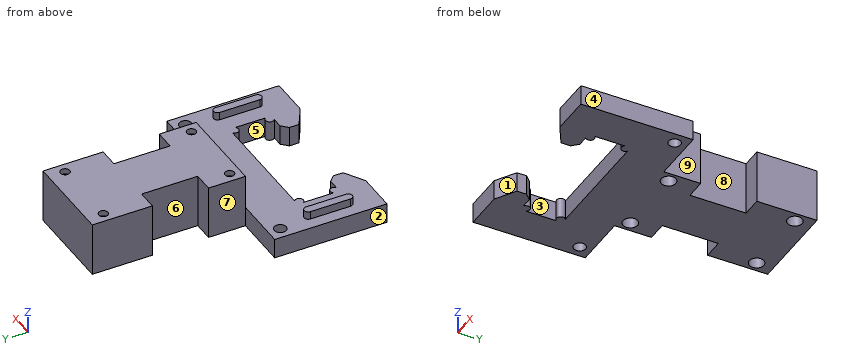
from build123d import *

# Parameters (mm, degrees)
ESQUISSE1_W             = 63.5
ESQUISSE1_H             = 35.56
BOSS_EXTRU_1_DEPTH      = 6.35
BOSS_EXTRU_2_DEPTH      = 2.54
EMPREINTE1_DEPTH        = 6.35
D_PLACER_LA_FACE2_DEPTH = 6.35
CHANFREIN1_SIZE         = 6.35
CHANFREIN1_SIZE2        = 3.81
CHANFREIN2_SIZE         = 6.35
CHANFREIN2_SIZE2        = 3.81
ESQUISSE3_W             = 29
ESQUISSE3_H             = 17.046330794
BOSS_EXTRU_3_DEPTH      = 48.514
ESQUISSE4_R             = 2.341041465
ENL_V_MAT_EXTRU_1_DEPTH = 15.24
ESQUISSE5_R             = 1.397
ESQUISSE5_W             = 6.35
ESQUISSE5_H             = 17.78
ENL_V_MAT_EXTRU_2_DEPTH = 78.134580407
D_GAGEMENT_M2_51_D      = 2.9
D_GAGEMENT_61_D         = 3.7973


# Read off the part's stored shape, not the designer's step: Empreinte1, Déplacer la face2
with BuildPart() as part:
    # Esquisse1 → Boss.-Extru.1 (new body)
    with BuildSketch(Plane.XY):
        with Locations((0, 1.905)):
            Rectangle(ESQUISSE1_W, ESQUISSE1_H)
    extrude(amount=BOSS_EXTRU_1_DEPTH)

    # Esquisse2 → Boss.-Extru.2 (add)
    with BuildSketch(Plane.XY.offset(6.35)):
        with BuildLine():
            Line((-27.94, -6.35), (-27.94, 6.35))
            ThreePointArc((-27.94, 6.35), (-26.67, 7.62), (-25.4, 6.35))
            Line((-25.4, 6.35), (-25.4, -6.35))
            ThreePointArc((-25.4, -6.35), (-26.67, -7.62), (-27.94, -6.35))
        make_face()
    boss_extru_2 = extrude(amount=BOSS_EXTRU_2_DEPTH)

    # Symétrie1: Boss.-Extru.2 across plane
    add(boss_extru_2.mirror(Plane(origin=(0, 0, 0), x_dir=(0, 0, 1), z_dir=(1, 0, 0))))

    # Empreinte1 outline → Empreinte1 (cut)
    with BuildSketch(Plane.XY):
        with BuildLine():
            Line((-11.90625, -8.5725), (-11.90625, -15.875))
            Line((-11.90625, -15.875), (11.90625, -15.875))
            Line((11.90625, -15.875), (11.90625, -8.5725))
            Line((11.90625, -8.5725), (14.44625, -6.0325))
            Line((14.44625, -6.0325), (16.66875, -6.0325))
            ThreePointArc((16.66875, -6.0325), (17.366201977, -4.348701977), (19.05, -3.65125))
            Line((19.05, -3.65125), (19.05, 2.69875))
            ThreePointArc((19.05, 2.69875), (17.366201977, 3.396201977), (16.66875, 5.08))
            Line((16.66875, 5.08), (-16.66875, 5.08))
            ThreePointArc((-16.66875, 5.08), (-17.366201977, 3.396201977), (-19.05, 2.69875))
            Line((-19.05, 2.69875), (-19.05, -3.65125))
            ThreePointArc((-19.05, -3.65125), (-17.366201977, -4.348701977), (-16.66875, -6.0325))
            Line((-16.66875, -6.0325), (-14.44625, -6.0325))
            Line((-14.44625, -6.0325), (-11.90625, -8.5725))
        make_face()
    extrude(amount=EMPREINTE1_DEPTH, mode=Mode.SUBTRACT)

    # Déplacer la face2 outline → Déplacer la face2 (cut)
    with BuildSketch(Plane.XY):
        with BuildLine():
            Line((-12.97305, -9.014383028), (-12.97305, -15.875))
            Line((-12.97305, -15.875), (-11.90625, -15.875))
            Line((-11.90625, -15.875), (-11.90625, -8.5725))
            Line((-11.90625, -8.5725), (-14.44625, -6.0325))
            Line((-14.44625, -6.0325), (-16.66875, -6.0325))
            ThreePointArc((-16.66875, -6.0325), (-17.366201977, -4.348701977), (-19.05, -3.65125))
            Line((-19.05, -3.65125), (-19.05, 2.69875))
            ThreePointArc((-19.05, 2.69875), (-17.366201977, 3.396201977), (-16.66875, 5.08))
            Line((-16.66875, 5.08), (16.66875, 5.08))
            ThreePointArc((16.66875, 5.08), (17.366201977, 3.396201977), (19.05, 2.69875))
            Line((19.05, 2.69875), (19.05, -3.65125))
            ThreePointArc((19.05, -3.65125), (17.366201977, -4.348701977), (16.66875, -6.0325))
            Line((16.66875, -6.0325), (14.44625, -6.0325))
            Line((14.44625, -6.0325), (11.90625, -8.5725))
            Line((11.90625, -8.5725), (11.90625, -15.875))
            Line((11.90625, -15.875), (12.97305, -15.875))
            Line((12.97305, -15.875), (12.97305, -9.014383028))
            Line((12.97305, -9.014383028), (14.888133028, -7.0993))
            Line((14.888133028, -7.0993), (18.282069949, -7.0993))
            ThreePointArc((18.282069949, -7.0993), (18.120543491, -5.103043491), (20.1168, -5.264569949))
            Line((20.1168, -5.264569949), (20.1168, 4.312069949))
            ThreePointArc((20.1168, 4.312069949), (18.120543491, 4.150543491), (18.282069949, 6.1468))
            Line((18.282069949, 6.1468), (-18.282069949, 6.1468))
            ThreePointArc((-18.282069949, 6.1468), (-18.120543491, 4.150543491), (-20.1168, 4.312069949))
            Line((-20.1168, 4.312069949), (-20.1168, -5.264569949))
            ThreePointArc((-20.1168, -5.264569949), (-18.120543491, -5.103043491), (-18.282069949, -7.0993))
            Line((-18.282069949, -7.0993), (-14.888133028, -7.0993))
            Line((-14.888133028, -7.0993), (-12.97305, -9.014383028))
        make_face()
    extrude(amount=D_PLACER_LA_FACE2_DEPTH, mode=Mode.SUBTRACT)

    # Chanfrein1
    chanfrein1_edges = [part.edges().sort_by_distance(p)[0] for p in [
        (12.97305, -15.875, 3.175),
    ]]
    chanfrein1_side = [part.faces().sort_by_distance(p)[0] for p in [
        (22.361525, -15.875, 3.175),
    ]]
    chamfer(chanfrein1_edges, length=CHANFREIN1_SIZE, length2=CHANFREIN1_SIZE2, reference=chanfrein1_side[0])

    # Chanfrein2
    chanfrein2_edges = [part.edges().sort_by_distance(p)[0] for p in [
        (-12.97305, -15.875, 3.175),
    ]]
    chanfrein2_side = [part.faces().sort_by_distance(p)[0] for p in [
        (-22.361525, -15.875, 3.175),
    ]]
    chamfer(chanfrein2_edges, length=CHANFREIN2_SIZE, length2=CHANFREIN2_SIZE2, reference=chanfrein2_side[0])

    # Esquisse3 → Boss.-Extru.3 (add)
    with BuildSketch(Plane(origin=(0, 19.685, 0), x_dir=(1, 0, 0), z_dir=(0, 1, 0))):
        with Locations((0, -8.523165397)):
            Rectangle(ESQUISSE3_W, ESQUISSE3_H)
    extrude(amount=BOSS_EXTRU_3_DEPTH)

    # Esquisse4 → Enlèv. mat.-Extru.1 (cut)
    with BuildSketch(Plane(origin=(0, 0, 0), x_dir=(-1, 0, 0), z_dir=(0, 0, -1))):
        with Locations((-11.25, 62.935)):
            Circle(ESQUISSE4_R)
        with Locations((11.25, 62.935)):
            Circle(ESQUISSE4_R)
        with Locations((11.25, 22.935)):
            Circle(ESQUISSE4_R)
        with Locations((-11.25, 22.935)):
            Circle(ESQUISSE4_R)
    extrude(amount=-ENL_V_MAT_EXTRU_1_DEPTH, mode=Mode.SUBTRACT)

    # Esquisse5 → Enlèv. mat.-Extru.2 (cut, through all)
    with BuildSketch(Plane(origin=(0, 0, 0), x_dir=(-1, 0, 0), z_dir=(0, 0, -1))):
        with Locations((-11.25, 22.935)):
            Circle(ESQUISSE5_R)
        with Locations((-11.25, 62.935)):
            Circle(ESQUISSE5_R)
        with Locations((11.25, 62.935)):
            Circle(ESQUISSE5_R)
        with Locations((11.25, 22.935)):
            Circle(ESQUISSE5_R)
        with Locations((11.325, 40.259)):
            Rectangle(ESQUISSE5_W, ESQUISSE5_H)
        with Locations((-11.325, 40.259)):
            Rectangle(ESQUISSE5_W, ESQUISSE5_H)
    extrude(amount=-ENL_V_MAT_EXTRU_2_DEPTH, mode=Mode.SUBTRACT)

    # Dégagement M2.51 (through all)
    with Locations(Plane(origin=(0, 0, 0), x_dir=(-1, 0, 0), z_dir=(0, 0, -1))):
        with Locations((11.25, 62.935), (-11.25, 62.935), (11.25, 22.935), (-11.25, 22.935)):
            Hole(D_GAGEMENT_M2_51_D / 2)

    # Dégagement #61 (through all)
    with Locations(Plane(origin=(0, 0, 0), x_dir=(-1, 0, 0), z_dir=(0, 0, -1))):
        with Locations((-27.94, 15.875), (27.94, 15.875)):
            Hole(D_GAGEMENT_61_D / 2)


solid = part.part
Design review of the part built by this model. Coordinates are the model's own, in mm. Face numbers are marked on the shaded views. A direction names the side the tool comes from. Coordinates: 2 decimals unless noted, no trailing zeros. Loops run counter-clockwise (first coordinate to the right, second up) from the corner with the lowest first, then second, coordinate; pieces in that order, holes last. Notation, with made-up numbers: M 46,66.25 L 73,66.25 A25 ccw 73,78.25 Z; hole C 30.5,-39 d10. An arc over 180 degrees is marked long. Answer as CSV lines item,"result".
Item 1: Add section B-B on x = -11.25. State the section outline as (y, z) points (3 decimals).
Answer list:
outline,"M 6.147,0 L 20.594,0 L 20.594,15.24 L 21.485,15.24 L 21.485,17.046 L 19.685,17.046 L 19.685,6.35 L 6.147,6.35 Z; M 24.385,15.24 L 25.276,15.24 L 25.276,0 L 31.369,0 L 31.369,17.046 L 24.385,17.046 Z; M 49.149,0 L 60.594,0 L 60.594,15.24 L 61.485,15.24 L 61.485,17.046 L 49.149,17.046 Z; M 64.385,15.24 L 65.276,15.24 L 65.276,0 L 68.199,0 L 68.199,17.046 L 64.385,17.046 Z"
Item 2: The part is to be moulded in two halves that separate along X. For the marked faces 1, 2, 3 and 4, say which applies: pulls with the +X half, pulls with the -X half, needs draft (parallel to the pull), parting line crosses it, or undercut.
Answer list:
face 1,"undercut"
face 2,"pulls with the -X half"
face 3,"undercut"
face 4,"pulls with the +X half"
Item 3: Add section D-D on z = 11.25. State the section outline as (x, y) points (3 decimals), plus the area to 3 significant figures.
Answer list:
outline,"M -14.5,19.685 L 14.5,19.685 L 14.5,31.369 L 8.15,31.369 L 8.15,49.149 L 14.5,49.149 L 14.5,68.199 L -14.5,68.199 L -14.5,49.149 L -8.15,49.149 L -8.15,31.369 L -14.5,31.369 Z; hole C -11.25,22.935 d4.682; hole C -11.25,62.935 d4.682; hole C 11.25,22.935 d4.682; hole C 11.25,62.935 d4.682"
area,"1,110 mm²"
Item 4: For probe 1 along Y at (x, z) = (11.25, 16.4) (3 decimals); probe 2 along Y at (x, z) = (-11.5, 13.25) (3 decimals); probe 3 along X at (y, z) = (64, 2), list the stretches that pass through material, from the lowest coordinate up.
Answer list:
probe 1,"19.685 to 21.485, 24.385 to 31.369, 49.149 to 61.485, 64.385 to 68.199"
probe 2,"19.685 to 20.607, 25.263 to 31.369, 49.149 to 60.607, 65.263 to 68.199"
probe 3,"-14.5 to -13.33, -9.17 to 9.17, 13.33 to 14.5"
Item 5: For P1, Ø10.5, axis at x = 3, y = -6.5, coming from the +Z side; P2, Ø3, axis at y = -3, z = 8, coming from the -X side; P3, Ø2.5, axis at x = 11, y = 22, coming from the -Z side; P4, Ø4, axis at x = -8, z = 11, coming from the -Y side (3 decimals), all flat-tipped, find the tip position at first contact; note any pin that passes through.
Answer list:
P1,"through"
P2,"x = -27.94"
P3,"z = 15.24"
P4,"y = 19.685"
Item 6: Add section A-A on y = 0.5. State the section outline as (x, z) points.
Answer list:
outline,"M -31.75,0 L -20.12,0 L -20.12,6.35 L -25.4,6.35 L -25.4,8.89 L -27.94,8.89 L -27.94,6.35 L -31.75,6.35 Z; M 20.12,0 L 31.75,0 L 31.75,6.35 L 27.94,6.35 L 27.94,8.89 L 25.4,8.89 L 25.4,6.35 L 20.12,6.35 Z"
Item 7: Machinability: for the marked faces 5, 6, 7, 8 and 9, which of the approach directions +Z, -Z, +X, -X, +Y, -Y give a long, thin tool a straight path to every point of the face, cutting with its end or side? Answer none if there is none.
Answer list:
face 5,"+Z, -Z"
face 6,"+Z, -Z, -X"
face 7,"+Z, -Z, -X, +Y"
face 8,"+Z, -Z, +X"
face 9,"+Z, -Z, +X, +Y"
Item 8: Add section C-C on z = 7.5. State the section outline as (x, y) points (3 decimals), plus the area to 3 significant figures.
Answer list:
outline,"M -27.94,-6.35 A1.27 ccw -25.4,-6.35 L -25.4,6.35 A1.27 ccw -27.94,6.35 Z; M -14.5,19.685 L 14.5,19.685 L 14.5,31.369 L 8.15,31.369 L 8.15,49.149 L 14.5,49.149 L 14.5,68.199 L -14.5,68.199 L -14.5,49.149 L -8.15,49.149 L -8.15,31.369 L -14.5,31.369 Z; M 25.4,-6.35 A1.27 ccw 27.94,-6.35 L 27.94,6.35 A1.27 ccw 25.4,6.35 Z; hole C -11.25,22.935 d4.682; hole C -11.25,62.935 d4.682; hole C 11.25,22.935 d4.682; hole C 11.25,62.935 d4.682"
area,"1,190 mm²"
